```python
from build123d import *

# Parameters (mm, degrees)
SKETCH1_R                   = 25.3365
BOSS_EXTRUDE1_DEPTH         = 2.54
SKETCH2_R                   = 23.241
BOSS_EXTRUDE2_DEPTH         = 2.54
F_1_4_CLEARANCE_HOLE1_D     = 6.5278
F_1_4_CLEARANCE_HOLE1_DEPTH = 5.08
CUT_EXTRUDE1_REACH          = 7.08
SKETCH5_R                   = 2.8575
CUT_EXTRUDE2_REACH          = 7.08
SKETCH6_R                   = 1.136382046


with BuildPart() as part:
    # Sketch1 → Boss-Extrude1 (new body)
    with BuildSketch(Plane(origin=(0, 0, 0), x_dir=(1, 0, 0), z_dir=(0, 1, 0))):
        Circle(SKETCH1_R)
    extrude(amount=BOSS_EXTRUDE1_DEPTH)

    # Sketch2 → Boss-Extrude2 (add)
    with BuildSketch(Plane(origin=(0, 2.54, 0), x_dir=(1, 0, 0), z_dir=(0, 1, 0))):
        Circle(SKETCH2_R)
    extrude(amount=BOSS_EXTRUDE2_DEPTH)

    # 1/4 Clearance Hole1
    with Locations(Plane.XZ):
        with Locations((0, 0)):
            Hole(F_1_4_CLEARANCE_HOLE1_D / 2, depth=F_1_4_CLEARANCE_HOLE1_DEPTH)

    # Sketch5 → Cut-Extrude1 (cut, up to next)
    with BuildSketch(Plane.XZ, mode=Mode.PRIVATE) as cut_extrude1_sk1:
        with Locations((-19.685, 0)):
            Circle(SKETCH5_R)
    cut_extrude1_tool1 = extrude(cut_extrude1_sk1.sketch, amount=-CUT_EXTRUDE1_REACH, mode=Mode.PRIVATE) & part.part
    add(cut_extrude1_tool1.solids().sort_by_distance((-19.685, 0, 0))[0], mode=Mode.SUBTRACT)
    # Sketch5 → Cut-Extrude1 (cut, up to next)
    with BuildSketch(Plane.XZ, mode=Mode.PRIVATE) as cut_extrude1_sk2:
        with Locations((19.685, 0)):
            Circle(SKETCH5_R)
    cut_extrude1_tool2 = extrude(cut_extrude1_sk2.sketch, amount=-CUT_EXTRUDE1_REACH, mode=Mode.PRIVATE) & part.part
    add(cut_extrude1_tool2.solids().sort_by_distance((19.685, 0, 0))[0], mode=Mode.SUBTRACT)

    # Sketch6 → Cut-Extrude2 (cut, up to next)
    with BuildSketch(Plane.XZ, mode=Mode.PRIVATE) as cut_extrude2_sk1:
        with Locations((-7.069885154, 12.643721498)):
            Circle(SKETCH6_R)
    cut_extrude2_tool1 = extrude(cut_extrude2_sk1.sketch, amount=-CUT_EXTRUDE2_REACH, mode=Mode.PRIVATE) & part.part
    add(cut_extrude2_tool1.solids().sort_by_distance((-7.069885, 0, 12.643721))[0], mode=Mode.SUBTRACT)
    # Sketch6 → Cut-Extrude2 (cut, up to next)
    with BuildSketch(Plane.XZ, mode=Mode.PRIVATE) as cut_extrude2_sk2:
        with Locations((-12.50848412, 7.306489885)):
            Circle(SKETCH6_R)
    cut_extrude2_tool2 = extrude(cut_extrude2_sk2.sketch, amount=-CUT_EXTRUDE2_REACH, mode=Mode.PRIVATE) & part.part
    add(cut_extrude2_tool2.solids().sort_by_distance((-12.508484, 0, 7.30649))[0], mode=Mode.SUBTRACT)


solid = part.part
```
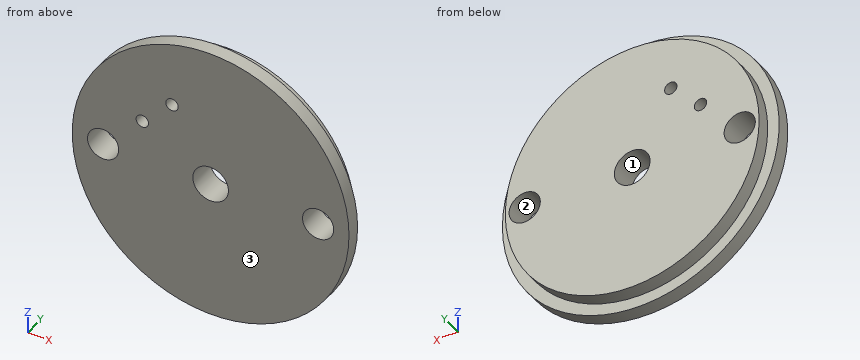
Geometry: final body of the model. Coordinates: model frame, mm. Face numbers are marked on the shaded views. Give positions to 0.01 mm unless a question says otherwise; leave off trailing zeros. Loops run counter-clockwise (first coordinate to the right, second up) from the corner with the lowest first, then second, coordinate; pieces in that order, holes last. Notation, with made-up numbers: (17.5, 43.5) -> (27.5, 43.5) arc R32 cw to (27.5, 81.5) -> close; hole circle Ø2 at (-40, 32.5). An arc over 180 degrees is marked (long way). Use CSV: the item, a comma, the result in double quotes.
(1) Cut plane C-C (y = 3.2). Output: boundary loops of the cut face in (x, z) (1 decimal).
From the geometry:
outline,"circle Ø46.5 at (0, 0); hole circle Ø5.7 at (-19.7, 0); hole circle Ø2.3 at (-12.5, 7.3); hole circle Ø2.3 at (-7.1, 12.6); hole circle Ø6.5 at (0, 0); hole circle Ø5.7 at (19.7, 0)"
(2) Ray query, line 1 along X through (y, z) = (1.95, -1); line 2 along Z through (x, y) = (0, 2.3); line 3 along Z through (x, y) = (-19.5, 3.85). Return the intervals inside material, ascending. Write a range as [from, to].
From the geometry:
line 1,"[-25.32, -22.36], [-17.01, -3.11], [3.11, 17.01], [22.36, 25.32]"
line 2,"[-25.34, -3.26], [3.26, 25.34]"
line 3,"[-12.64, -2.85], [2.85, 12.64]"
(3) Cut plane D-D (x = -12). Output: boundary loops of the cut face in (y, z), plus the area to 3 significant figures.
From the geometry:
outline,"(0, -22.31) -> (2.54, -22.31) -> (2.54, -19.9) -> (5.08, -19.9) -> (5.08, 6.29) -> (0, 6.29) -> close; (0, 8.32) -> (5.08, 8.32) -> (5.08, 19.9) -> (2.54, 19.9) -> (2.54, 22.31) -> (0, 22.31) -> close"
area,"204 mm^2"
(4) First-contact query: P1, Ø2, axis at x = -12.51, z = 7.31, coming from the -Y side (1 decimal); P2, Ø1.5, axis at x = 17.5, y = 3, coming from the -Z side. Flat tips, straight axial feed; report the tip coordinate or a pass-through.
From the geometry:
P1,"through"
P2,"z = -18.87"
(5) Cut plane A-A (x = 0). Output: boundary loops of the cut face in (y, z), plus the area to 3 significant figures.
From the geometry:
outline,"(0, -25.34) -> (2.54, -25.34) -> (2.54, -23.24) -> (5.08, -23.24) -> (5.08, -3.26) -> (0, -3.26) -> close; (0, 3.26) -> (5.08, 3.26) -> (5.08, 23.24) -> (2.54, 23.24) -> (2.54, 25.34) -> (0, 25.34) -> close"
area,"214 mm^2"
(6) Cut plane B-B (z = 0). Output: boundary loops of the cut face in (x, y).
From the geometry:
outline,"(-25.34, 0) -> (-22.54, 0) -> (-22.54, 5.08) -> (-23.24, 5.08) -> (-23.24, 2.54) -> (-25.34, 2.54) -> close; (-16.83, 0) -> (-3.26, 0) -> (-3.26, 5.08) -> (-16.83, 5.08) -> close; (3.26, 0) -> (16.83, 0) -> (16.83, 5.08) -> (3.26, 5.08) -> close; (22.54, 0) -> (25.34, 0) -> (25.34, 2.54) -> (23.24, 2.54) -> (23.24, 5.08) -> (22.54, 5.08) -> close"
(7) Pull-direction query (Z, two-part tool) for the marked faces 1, 2 and 3; classes: released by +Z, released by -Z, zero draft, split by the parting line, or undercut.
From the geometry:
face 1,"undercut"
face 2,"undercut"
face 3,"zero draft"
